Geometry: final body of the model. Coordinates: model frame, mm. Face numbers are marked on the shaded views. A direction names the side the tool comes from. Give positions to 0.01 mm unless a question says otherwise; leave off trailing zeros. Loops run counter-clockwise (first coordinate to the right, second up) from the corner with the lowest first, then second, coordinate; pieces in that order, holes last. Notation, with made-up numbers: (52, 5) - (78, 5) arc R30 cw to (78, 31) - close; hole circle Ø8 at (87, 40). An arc over 180 degrees is marked (long way). Use one line per item in the form item = value.
```python
from build123d import *

# Parameters (mm, degrees)
SKETCH1_W            = 22.7838
SKETCH1_H            = 11.6332
BOSS_EXTRUDE1_DEPTH  = 15.9512
FILLET1_R            = 0.508
BOSS_EXTRUDE3_DEPTH  = 11.6332
CUT_EXTRUDE1_DEPTH   = 4.0132
CHAMFER1_SIZE        = 0.127
FILLET2_R            = 1.016
SKETCH7_R            = 2.0066
CUT_EXTRUDE2_DEPTH   = 18.9197
BOSS_EXTRUDE4_DEPTH  = 2.794
SKETCH9_R            = 2.794
CUT_EXTRUDE3_DEPTH   = 0.254
BOSS_EXTRUDE5_DEPTH  = 1.016
BOSS_EXTRUDE6_DEPTH  = 1.016
SKETCH12_R           = 2.2479
SKETCH12_R_2         = 0.9906
BOSS_EXTRUDE10_DEPTH = 3.3782
FILLET3_R            = 0.1016


with BuildPart() as part:
    # Sketch1 → Boss-Extrude1 (new body)
    with BuildSketch(Plane(origin=(0, 0, 0), x_dir=(1, 0, 0), z_dir=(0, 1, 0))):
        with Locations((-11.3919, -5.8166)):
            Rectangle(SKETCH1_W, SKETCH1_H)
    extrude(amount=BOSS_EXTRUDE1_DEPTH)

    # Fillet1
    fillet1_edges = [part.edges().sort_by_distance(p)[0] for p in [
        (-11.3919, 0, 11.6332),
        (-22.7838, 0, 5.8166),
        (-11.3919, 0, 0),
        (0, 0, 5.8166),
    ]]
    fillet(fillet1_edges, radius=FILLET1_R)

    # Sketch5 → Boss-Extrude3 (add)
    with BuildSketch(Plane.XY.offset(11.6332)):
        Polygon((0, 15.9512), (4.9784, 15.9512), (4.9784, 17.9197), (0, 17.9197), (0, 20.4597), (-5.9436, 22.2504), (-7.512738225, 22.2504), (-7.512738225, 26.2636), (-22.7838, 26.2636), (-22.7838, 17.9197), (-27.7622, 17.9197), (-27.7622, 15.9512), (-22.7838, 15.9512), align=None)
    extrude(amount=-BOSS_EXTRUDE3_DEPTH)

    # Sketch6 → Cut-Extrude1 (cut)
    with BuildSketch(Plane(origin=(0, 26.2636, 0), x_dir=(1, 0, 0), z_dir=(0, 1, 0))):
        with BuildLine():
            Line((-18.93048198, 0), (-22.7838, 0))
            Line((-22.7838, 0), (-22.7838, -11.6332))
            Line((-22.7838, -11.6332), (-18.93048198, -11.6332))
            ThreePointArc((-18.93048198, -11.6332), (-22.733, -5.8166), (-18.93048198, 0))
        make_face()
        with BuildLine():
            Line((-7.512738225, 0), (-13.83551802, 0))
            ThreePointArc((-13.83551802, 0), (-11.067973632, -2.341978479), (-10.033, -5.8166))
            ThreePointArc((-10.033, -5.8166), (-11.067973632, -9.291221521), (-13.83551802, -11.6332))
            Line((-13.83551802, -11.6332), (-7.512738225, -11.6332))
            Line((-7.512738225, -11.6332), (-7.512738225, 0))
        make_face()
    extrude(amount=-CUT_EXTRUDE1_DEPTH, mode=Mode.SUBTRACT)

    # Chamfer1
    chamfer1_edges = [part.edges().sort_by_distance(p)[0] for p in [
        (-16.383, 26.2636, 11.6332),
        (-22.733, 26.2636, 5.8166),
        (-16.383, 26.2636, 0),
        (-10.033, 26.2636, 5.8166),
    ]]
    chamfer(chamfer1_edges, length=CHAMFER1_SIZE)

    # Fillet2
    fillet2_edges = [part.edges().sort_by_distance(p)[0] for p in [
        (-27.7622, 16.93545, 0),
        (-27.7622, 16.93545, 11.6332),
        (4.9784, 16.93545, 0),
        (4.9784, 16.93545, 11.6332),
    ]]
    fillet(fillet2_edges, radius=FILLET2_R)

    # Sketch7 → Cut-Extrude2 (cut, through all)
    with BuildSketch(Plane(origin=(0, 17.9197, 0), x_dir=(1, 0, 0), z_dir=(0, 1, 0))):
        with Locations((3.4671, -5.8166)):
            Circle(SKETCH7_R)
        with Locations((-26.2509, -5.8166)):
            Circle(SKETCH7_R)
    extrude(amount=-CUT_EXTRUDE2_DEPTH, mode=Mode.SUBTRACT)

    # Sketch8 → Boss-Extrude4 (add)
    with BuildSketch(Plane(origin=(0, 22.2504, 0), x_dir=(1, 0, 0), z_dir=(0, 1, 0))):
        with BuildLine():
            Line((-7.679090009, -2.88804007), (-13.538580336, -0.139296346))
            ThreePointArc((-13.538580336, -0.139296346), (-10.033, -5.8166), (-13.538580336, -11.493903654))
            Line((-13.538580336, -11.493903654), (-7.679090009, -8.74515993))
            ThreePointArc((-7.679090009, -8.74515993), (-6.704959334, -7.430304447), (-6.433420255, -5.8166))
            ThreePointArc((-6.433420255, -5.8166), (-6.704959334, -4.202895553), (-7.679090009, -2.88804007))
        make_face()
    extrude(amount=BOSS_EXTRUDE4_DEPTH)

    # Sketch9 → Cut-Extrude3 (cut)
    with BuildSketch(Plane(origin=(0, 26.2636, 0), x_dir=(1, 0, 0), z_dir=(0, 1, 0))):
        with Locations((-16.383, -5.8166)):
            Circle(SKETCH9_R)
    extrude(amount=-CUT_EXTRUDE3_DEPTH, mode=Mode.SUBTRACT)

    # Sketch10 → Boss-Extrude5 (add)
    with BuildSketch(Plane.XY.offset(11.6332)):
        Polygon((0, 20.2565), (3.175, 17.9197), (0, 17.9197), align=None)
        Polygon((-22.7838, 17.9197), (-22.7838, 20.2565), (-25.9588, 17.9197), align=None)
    extrude(amount=-BOSS_EXTRUDE5_DEPTH)

    # Sketch11 → Boss-Extrude6 (add)
    with BuildSketch(Plane(origin=(0, 0, 0), x_dir=(-1, 0, 0), z_dir=(0, 0, -1))):
        Polygon((22.7838, 20.2565), (22.7838, 17.9197), (25.9588, 17.9197), align=None)
        Polygon((0, 20.2565), (-3.175, 17.9197), (0, 17.9197), align=None)
    extrude(amount=-BOSS_EXTRUDE6_DEPTH)

    # Sketch12 → Boss-Extrude10 (add)
    with BuildSketch(Plane(origin=(0, 26.0096, 0), x_dir=(1, 0, 0), z_dir=(0, 1, 0))):
        with Locations((-16.383, -5.8166)):
            Circle(SKETCH12_R)
        with Locations((-16.383, -5.8166)):
            Circle(SKETCH12_R_2, mode=Mode.SUBTRACT)
    extrude(amount=BOSS_EXTRUDE10_DEPTH)

    # Fillet3
    fillet3_edges = [part.edges().sort_by_distance(p)[0] for p in [
        (-18.6309, 29.3878, 5.8166),
    ]]
    fillet(fillet3_edges, radius=FILLET3_R)


solid = part.part
```
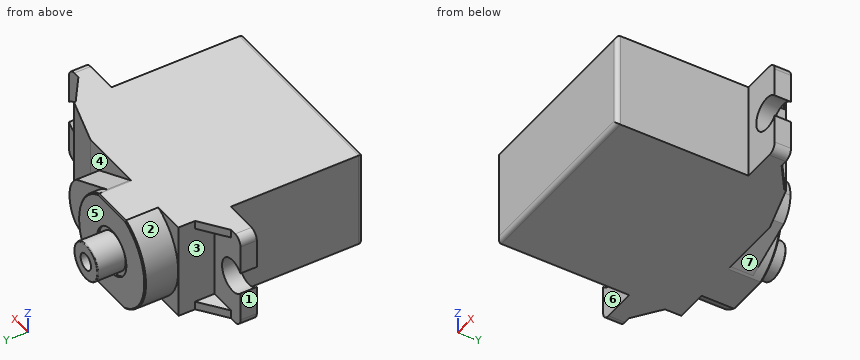
(1) Cut plane B-B (y = 25.5). Return the cut outline in (x, z), plus the area to 3 significant figures.
Solution:
outline = (-18.93, 0) - (-13.84, 0) arc R6.35 ccw to (-13.84, 11.63) - (-18.93, 11.63) arc R6.35 ccw to start
area = 123 mm2
(2) Cut plane C-C (y = 15). Return the cut outline in (x, z), plus the area to 3 significant figures.
Solution:
outline = (-22.78, 0) - (0, 0) - (0, 11.63) - (-22.78, 11.63) - close
area = 265 mm2
(3) Access query for the marked faces 4, 5, 6 and 7. Directions: +Z, -Z, +X, -X, +Y, -Y. A direction counts if a zero-diameter tool reaches every point of the face in a straight line with its end or side. Return the directions, or none.
Solution:
face_4 = +X, +Y
face_5 = +Y
face_6 = +Z, -Z, -X, -Y
face_7 = -Z, +X, +Y
(4) Pull-direction query (Z, two-part tool) for the marked faces 1, 2 and 3; classes: released by +Z, released by -Z, zero draft, split by the parting line, or undercut.
Solution:
face_1 = zero draft
face_2 = split by the parting line
face_3 = undercut
(5) Cut plane D-D (x = -5). Return the cut outline in (y, z), plus the area to 3 significant figures.
Solution:
outline = (0, 0.51) arc R0.51 ccw to (0.51, 0) - (21.97, 0) - (21.97, 11.63) - (0.51, 11.63) arc R0.51 ccw to (0, 11.13) - close
area = 255 mm2
(6) Cut plane A-A (x = 0.5). Return the cut outline in (y, z).
Solution:
outline = (15.95, 0) - (19.89, 0) - (19.89, 1.02) - (17.92, 1.02) - (17.92, 10.62) - (19.89, 10.62) - (19.89, 11.63) - (15.95, 11.63) - close
(7) Pin query (flat end, axial travel): P1, Ø1.9, axis at x = -25, y = 19.5, coming from the -Z side; P2, Ø1, axis at x = -16.5, z = 6, coming from the +Y side; P3, Ø4.5, axis at x = 3.47, z = 5.82, coming from the +Y side; P4, Ø6, axis at y = 6.5, z = 3, coming from the -X side. Return the tip coordinate at first contact, or that it passes through.
Solution:
P1 = 0
P2 = 26.01
P3 = 17.92
P4 = -22.78
(8) Material intervals for L1, parallel to X at y = 11, z = 7; L2, parallel to Y at x = -17, z = 2.25; L3, parallel to Y at x = -23.5, z = 2.25, sorted ascending. Write a range as from..to.
Solution:
L1 = -22.78..0
L2 = 0..26.26
L3 = 15.95..17.92
